Design review of the part shown in the three views and the two pictorial views. Dimensions are in mm from the part's minimum x, y and z. A direction names the side the tool comes from. Coordinates: 2 decimals unless noted, no trailing zeros. Loops run counter-clockwise (first coordinate to the right, second up) from the corner with the lowest first, then second, coordinate; pieces in that order, holes last. Notation, with made-up numbers: (81.5, 12.5) -> (134.5, 12.5) arc R21 cw to (134.5, 40.5) -> close; hole circle Ø5 at (64.25, 73.25). An arc over 180 degrees is marked (long way). Use a Markdown table: item, result. Add a question column.
Q1. Take a section at A-A on z = 9. Write out the cut boundary in (x, y) (1 decimal), plus the area to 3 significant figures.
Q2. Take a section at C-C on x = 33. Write out the cut boundary in (y, z).
Q3. Take a section at B-B on y = 4. Write out the cut boundary in (x, z).
Q4. Clearance check with flat-ended pins moving along their axes: pin 1 Ø3 at (y, z) = (63, 5.5) entering from +X; pin 2 Ø1.2 at (x, z) = (55.5, 5.5) entering from +Y (1 decimal); pin 3 Ø1.3 at (y, z) = (62, 10) entering from -X. State where each tip first meets the part, or that it passes through.
Q5. For probe 1 along Z at (x, y) = (33, 51.25); probe 2 along X at (y, z) = (23, 14); probe 3 along X at (y, z) = (10, 17.25), list the stretches that pass through material, from the lowest coordinate up.
Q6. Draft analysis for pull direction Y (two halves, no side actions). For the marked faces 4, 5, 6 and 7, state which applies: pulls with the +Y half, pulls with the -Y half, needs draft (parallel to the pull), parting line crosses it, or undercut.
Q7. Take a section at D-D on z = 16.5. Write out the cut boundary in (x, y) (1 decimal), plus the area to 3 significant figures.
Q8. For the marked faces 1, 2 and 3, list the 3-axis set-ups (+Z, -Z, +X, -X, +Y, -Y) from which the entire face can be reached by the end or side of a thin tool; tool diameter is ignored.
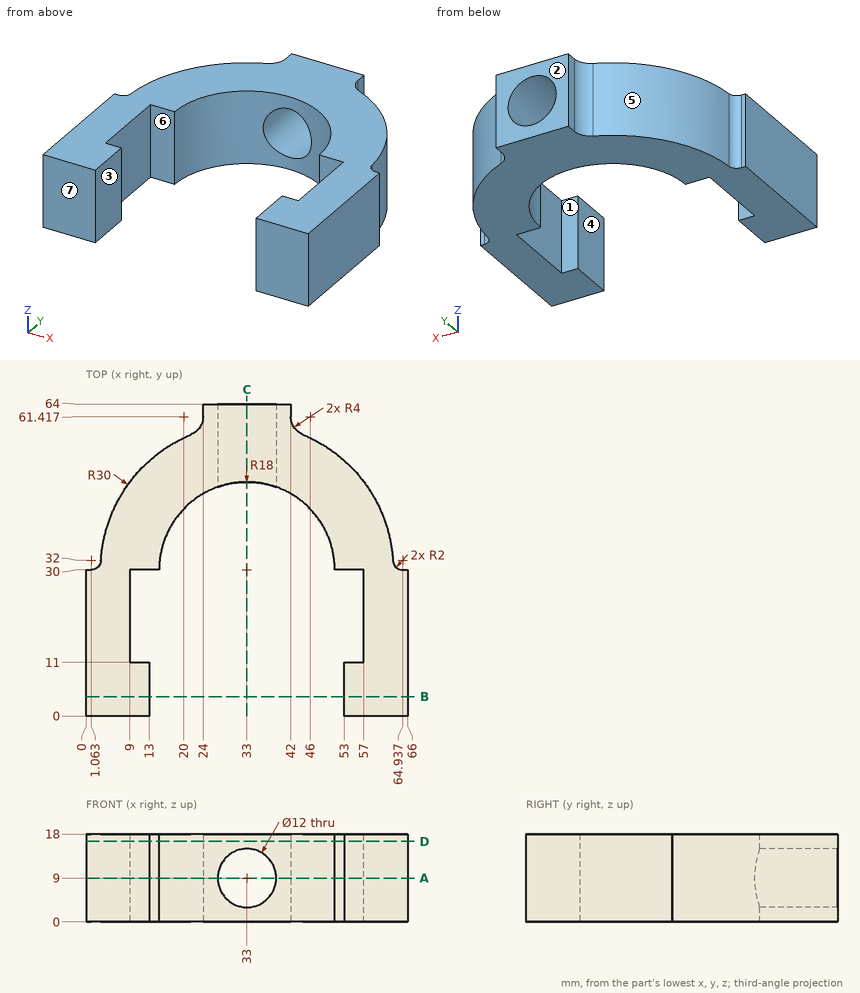
Answer list:
| question | item | result |
|---|---|---|
| 1 | outline | (0, 0) -> (13, 0) -> (13, 11) -> (9, 11) -> (9, 30) -> (15, 30) arc R18 cw to (27, 47) -> (27, 64) -> (24, 64) -> (24, 61.4) arc R4 cw to (21.5, 57.7) arc R30 ccw to (3.1, 31.9) arc R2 cw to (1.1, 30) -> (0, 30) -> close; (39, 47) arc R18 cw to (51, 30) -> (57, 30) -> (57, 11) -> (53, 11) -> (53, 0) -> (66, 0) -> (66, 30) -> (64.9, 30) arc R2 cw to (62.9, 31.9) arc R30 ccw to (44.5, 57.7) arc R4 cw to (42, 61.4) -> (42, 64) -> (39, 64) -> close |
| 1 | area | 1,420 mm² |
| 2 | outline | (48, 0) -> (64, 0) -> (64, 3) -> (48, 3) -> close; (48, 15) -> (64, 15) -> (64, 18) -> (48, 18) -> close |
| 3 | outline | (0, 0) -> (13, 0) -> (13, 18) -> (0, 18) -> close; (53, 0) -> (66, 0) -> (66, 18) -> (53, 18) -> close |
| 4 | pin 1 | x = 42 |
| 4 | pin 2 | y = 50.5 |
| 4 | pin 3 | x = 24 |
| 5 | probe 1 | 0 to 3, 15 to 18 |
| 5 | probe 2 | 0 to 9, 57 to 66 |
| 5 | probe 3 | 0 to 13, 53 to 66 |
| 6 | face 4 | needs draft |
| 6 | face 5 | pulls with the +Y half |
| 6 | face 6 | undercut |
| 6 | face 7 | pulls with the -Y half |
| 7 | outline | (0, 0) -> (13, 0) -> (13, 11) -> (9, 11) -> (9, 30) -> (15, 30) arc R18 cw to (51, 30) -> (57, 30) -> (57, 11) -> (53, 11) -> (53, 0) -> (66, 0) -> (66, 30) -> (64.9, 30) arc R2 cw to (62.9, 31.9) arc R30 ccw to (44.5, 57.7) arc R4 cw to (42, 61.4) -> (42, 64) -> (24, 64) -> (24, 61.4) arc R4 cw to (21.5, 57.7) arc R30 ccw to (3.1, 31.9) arc R2 cw to (1.1, 30) -> (0, 30) -> close |
| 7 | area | 1,620 mm² |
| 8 | face 1 | +Z, -Z |
| 8 | face 2 | +Z, -Z, +X, -X, +Y |
| 8 | face 3 | +Z, -Z, -Y |
